Part print with two shaded views. Sizes in mm from the minimum x, y, z corner. A direction names the side the tool comes from. Round coordinates to 2 decimals unless told otherwise and drop trailing zeros. Order: outer loops, then holes, each group sorted by start corner. A loop starts at its lowest first (then second) coordinate and runs counter-clockwise, first axis right, second up. Notation, with made-up numbers: (26.25, -0.75) -> (78.25, -0.75) arc R37 ccw to (78.25, 38.25) -> close; hole circle Ø10 at (-28, -16.75). An arc over 180 degrees is marked (long way). Put each result on its own line as item: value. Start each with the question number.
Q1. 3-axis set-ups, long thin cutter, end or side, ignore diameter. For the marked faces 4 and 5: which of +Z, -Z, +X, -X, +Y, -Y reach the whole face in a straight line?
Q2. Cut at C-C, the plane z = 40. List the corners of the cut face in (x, y) (1 decimal), and give its area (3 significant figures).
Q3. Cut at A-A, the plane x = 50.8. List the corners of the cut face in (y, z).
Q4. Cut at B-B, the plane y = 63.5. List the corners of the cut face in (x, z).
Q5. Pull direction Z, two halves, no side cores. Call the marked faces 1, 2 and 3: released by +Z, released by -Z, zero draft, split by the parting line, or undercut.
Q6. Flat gauge pins, fed straight in: P1, Ø12, axis at y = 67.5, z = 61, coming from the +X side; P2, Ø12, axis at x = 132.5, z = 82.5, coming from the -Y side; P3, Ø12.5, axis at y = 59.5, z = 37.5, coming from the +X side; P4, Ø7.5, axis at x = 117.5, y = 63, coming from the +Z side. Where does each tip first touch, or does it go through?
Q7. Probe L1, parallel to Z at x = 50, y = 17; L2, parallel to X at y = 18, z = 50; L3, parallel to Z at x = 69.5, y = 40. List the from-to ranges inside material, lowest first.
Q8. Cut at D-D, the plane z = 91. List the corners of the cut face in (x, y), and give its area (3 significant figures).
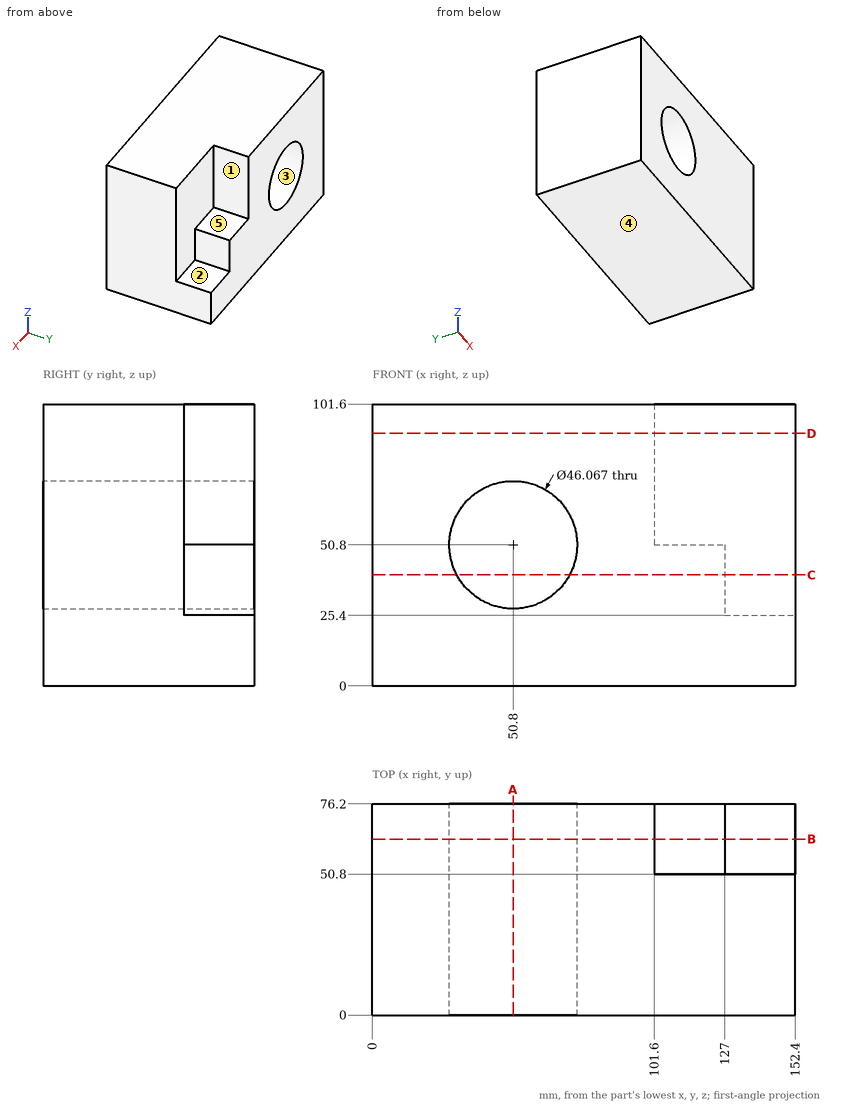
Ans:
1. face 4: -Z, +X, -X, +Y, -Y
1. face 5: +Z, +X, +Y
2. outline: (0, 0) -> (30.5, 0) -> (30.5, 76.2) -> (0, 76.2) -> close; (71.1, 0) -> (152.4, 0) -> (152.4, 50.8) -> (127, 50.8) -> (127, 76.2) -> (71.1, 76.2) -> close
2. area: 7,870 mm^2
3. outline: (0, 0) -> (76.2, 0) -> (76.2, 27.77) -> (0, 27.77) -> close; (0, 73.83) -> (76.2, 73.83) -> (76.2, 101.6) -> (0, 101.6) -> close
4. outline: (0, 0) -> (152.4, 0) -> (152.4, 25.4) -> (127, 25.4) -> (127, 50.8) -> (101.6, 50.8) -> (101.6, 101.6) -> (0, 101.6) -> close; hole circle Ø46.07 at (50.8, 50.8)
5. face 1: zero draft
5. face 2: released by +Z
5. face 3: undercut
6. P1: stops at x = 101.6
6. P2: stops at y = 0
6. P3: stops at x = 127
6. P4: stops at z = 50.8
7. L1: z = 0 to 27.78, 73.82 to 101.6
7. L2: x = 0 to 27.78, 73.82 to 152.4
7. L3: z = 0 to 37.35, 64.25 to 101.6
8. outline: (0, 0) -> (152.4, 0) -> (152.4, 50.8) -> (101.6, 50.8) -> (101.6, 76.2) -> (0, 76.2) -> close
8. area: 10,300 mm^2
